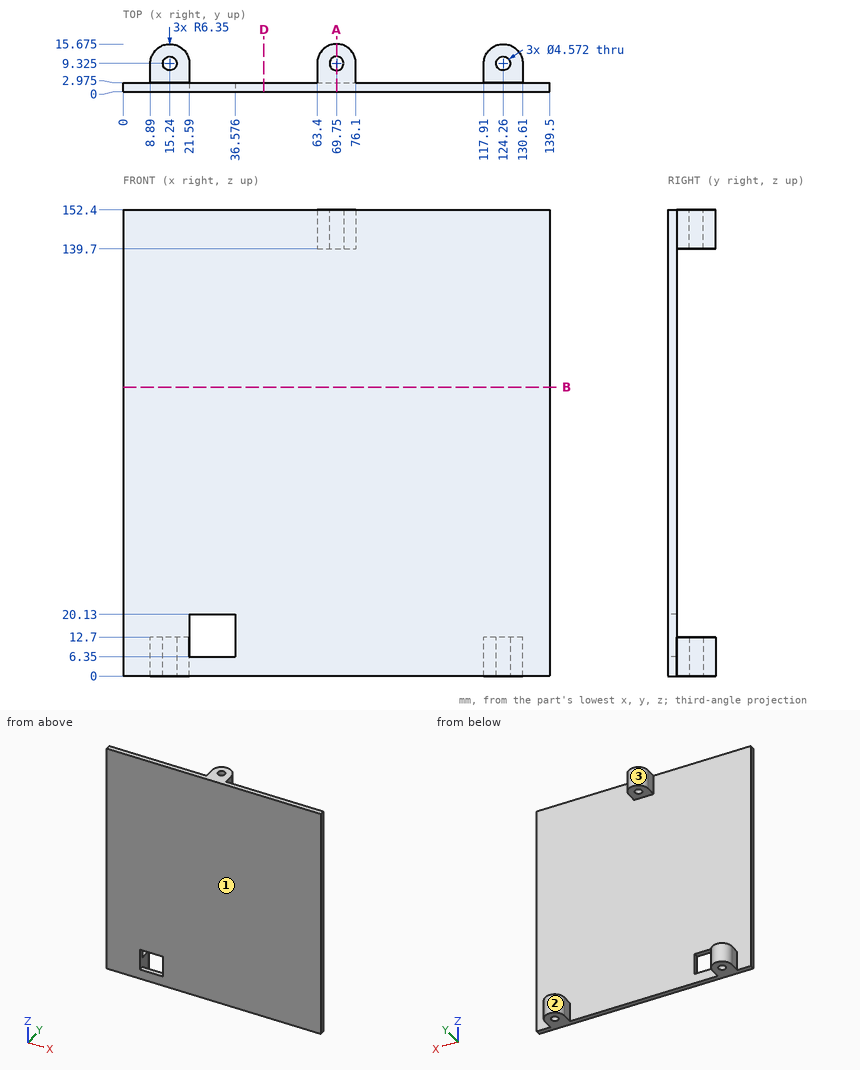
The drawing under review shows one solid part. Ordinate dimensions are in mm from its lowest x, y, z. Round coordinates to 2 decimals unless told otherwise and drop trailing zeros. Write each loop counter-clockwise with the first axis right and the second up, starting at its lowest first coordinate (ties: lowest second). Pieces come first, ordered by that corner, then holes. Notation, with made-up numbers: (26, -16.5) -> (39, -16.5) arc R18 ccw to (39, 1.5) -> close; hole circle Ø7 at (-14.75, 56). An arc over 180 degrees is marked (long way). Put each result on its own line as item: value.
Q1. Consider section B-B on z = 94.5. State the section outline as (x, y) points (1 decimal), and give its area (3 significant figures).
Determined:
outline: (0, 0) -> (139.5, 0) -> (139.5, 3) -> (0, 3) -> close
area: 415 mm^2
Q2. Consider section A-A on x = 69.75. State the section outline as (y, z) points (1 decimal).
Determined:
outline: (0, 0) -> (3, 0) -> (3, 139.7) -> (7, 139.7) -> (7, 152.4) -> (0, 152.4) -> close; (11.6, 139.7) -> (15.7, 139.7) -> (15.7, 152.4) -> (11.6, 152.4) -> close
Q3. Clearance check with flat-ended pins moving along their axes: pin 1 Ø1.5 at (y, z) = (5.5, 24.5) entering from -X; pin 2 Ø6.5 at (x, y) = (69, 10.5) entering from -Z; pin 3 Ø6.5 at (x, y) = (126.5, 10.5) entering from +Z; pin 4 Ø5 at (y, z) = (7, 6) entering from -X. State where each tip first meets the part, or that it passes through.
Determined:
pin 1: passes through
pin 2: stops at z = 139.7
pin 3: stops at z = 12.7
pin 4: stops at x = 8.89
Q4. Consider section D-D on x = 46. State the section outline as (y, z) points (1 decimal).
Determined:
outline: (0, 0) -> (3, 0) -> (3, 152.4) -> (0, 152.4) -> close
Q5. To check wall thickness, follow L1, parallel to Y at x = 124.26, z = 4.25 (1 decimal); L2, parallel to Y at x = 72, z = 92 (1 decimal); L3, parallel to Y at x = 127.5, z = 7.5 (1 decimal). State the ranges of each line that lie inside material, in increasing order. Write a range as [from, to].
Determined:
L1: y = [0, 7], [11.6, 15.7]
L2: y = [0, 3]
L3: y = [0, 14.8]
Q6. The part is to be moulded in two halves that separate along X. For the marked faces 1, 2 and 3, say which applies: released by +X, released by -X, zero draft, split by the parting line, or undercut.
Determined:
face 1: zero draft
face 2: undercut
face 3: split by the parting line
